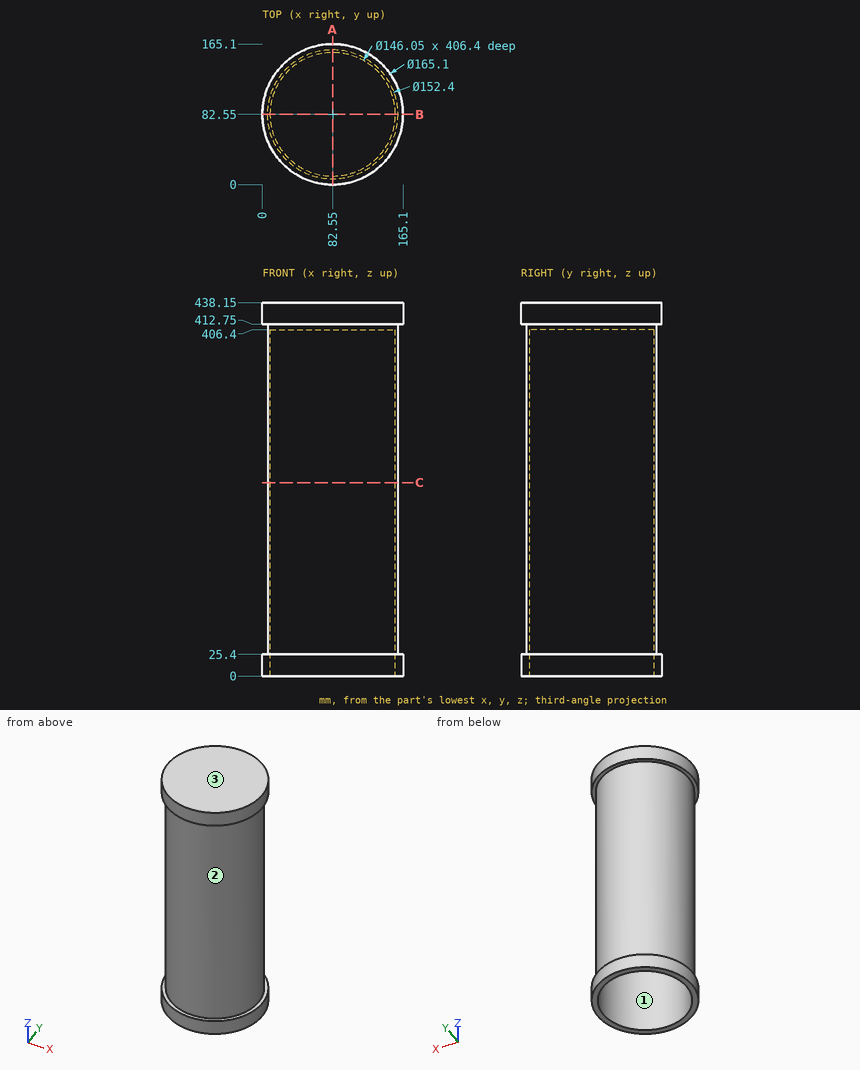
Geometry check sheet. Reference: drawing and pictorial views, mm from the part's lowest x, y, z. Give positions to 0.01 mm unless a question says otherwise; leave off trailing zeros. Order: outer loops, then holes, each group sorted by start corner. A loop starts at its lowest first (then second) coordinate and runs counter-clockwise, first axis right, second up. Notation, with made-up numbers: M 10,71 L 36,71 A26 cw 36,93 Z; hole C 39.5,43.5 d8. An arc over 180 degrees is marked long. Answer as a JSON object with one key per item and string values. Group by question number.
1) Cross-section at A-A (x = 82.55). Enter the section's corners in (y, z) (3 decimals), then the cut area to 3 significant figures.
2) Scan lines: line 1 along Y through (x, z) = (82.55, 129.5) (3 decimals); line 2 along X through (y, z) = (82, 271); line 3 along Z through (x, y) = (59.5, 29). Record each from-to range of solid material in increasing order. Write a range as [from, to].
3) Cross-section at C-C (z = 227). Enter the section's corners in (x, y) (3 decimals).
4) Depth check by flat-ended pin: pin 1 Ø2 at (x, y) = (142, 35) entering from -Z; pin 2 Ø1.5 at (x, z) = (108, 379) entering from -Y; pin 3 Ø2 at (y, z) = (61.5, 217) entering from -X; pin 4 Ø5 at (x, z) = (124.5, 331.5) entering from +Y. Enter the tip coordinate at first touch or a pass-through.
5) Mould release check, pull along Z, two halves, no side actions. Record for the marked faces 1, 2 and 3: released by +Z, released by -Z, zero draft, split by the parting line, or undercut.
Result sheet:
{
 "1": {"outline": "M 0,0 L 9.525,0 L 9.525,406.4 L 155.575,406.4 L 155.575,0 L 165.1,0 L 165.1,25.4 L 158.75,25.4 L 158.75,412.75 L 165.1,412.75 L 165.1,438.15 L 0,438.15 L 0,412.75 L 6.35,412.75 L 6.35,25.4 L 0,25.4 Z", "area": "8,060 mm2"},
 "2": {"line 1": "y = [6.35, 9.525], [155.575, 158.75]", "line 2": "x = [6.35, 9.53], [155.57, 158.75]", "line 3": "z = [406.4, 438.15]"},
 "3": {"outline": "C 82.55,82.55 d152.4; hole C 82.55,82.55 d146.05"},
 "4": {"pin 1": "stops at z = 0", "pin 2": "stops at y = 10.46", "pin 3": "stops at x = 9.04", "pin 4": "stops at y = 147.74"},
 "5": {"face 1": "zero draft", "face 2": "undercut", "face 3": "released by +Z"}
}
